Build history of the part. All positions in model axes, mm. A direction names the side the tool comes from. Round coordinates to 2 decimals unless told otherwise and drop trailing zeros. Loops run counter-clockwise (first coordinate to the right, second up) from the corner with the lowest first, then second, coordinate; pieces in that order, holes last. Notation, with made-up numbers: (-16, 58) -> (34, 58) arc R10 cw to (34, 72) -> close; hole circle Ø6 at (1, 37.25). An arc over 180 degrees is marked (long way). Put each result on its own line as item: value. Start each with the question number.
Item 1: Cut at C-C, the plane x = -4. List the corners of the cut face in (y, z) (3 decimals).
Item 2: Flat gauge pins, fed straight in: pin 1 Ø12 at (x, z) = (-22, -19.5) entering from -Y; pin 2 Ø0.5 at (y, z) = (0.5, -36.5) entering from +X; pin 3 Ø7.5 at (x, z) = (-12, -15.5) entering from +Y. Where does each tip first touch, or does it go through?
Item 3: Drill centre lines: probe 1 along X at (y, z) = (1, -55) (3 decimals); probe 2 along X at (y, z) = (4, -47.41); probe 3 along Z at (x, y) = (-11.5, 0.6) (3 decimals). Where is each one in solid material? Low to high. Write a range as [from, to].
Item 4: Cut at A-A, the plane y = 1.05. List the corners of the cut face in (x, z) (3 decimals).
Item 5: Tool access for faces 1 (the cylindrical face through (-18.156, 4.053, -35.451)), 2 (the flat face through (0, 2, -32)), 3 (the flat face through (-2.915, 1, -36)): list every direction of +Z, -Z, +X, -X, +Y, -Y with a clear straight run to the whole face (end or side of a thin tool).
Item 6: Cut at D-D, the plane x = -15.5. List the corners of the cut face in (y, z) (3 decimals), plus the area to 3 significant figures.
Item 7: Pull direction X, two halves, no side cores. Call faces 4 (the flat face through (-31, 2, -32)), 5 (the flat face through (-15, 2, 0)), 6 (the cylindrical face through (-3.044, 4.053, -20.09)): +X half, -X half, draft (parallel to the pull), parting line (faces both ways), or undercut.
Item 8: Cut at B-B, the plane z = -44. List the corners of the cut face in (x, y) (3 decimals).
Autodesk Inventor part; units mm, degrees
ref_plane "YZ Plane" through (0, 0, 0) normal (1, 0, 0) x (0, 1, 0)
ref_plane "XZ Plane" through (0, 0, 0) normal (0, 1, 0) x (-1, 0, 0)
ref_plane "XY Plane" through (0, 0, 0) normal (0, 0, 1) x (1, 0, 0)
sketch "Sketch1" plane through (0, 0, 0) normal (0, 1, 0) x (-1, 0, 0)
  line L0 (0, 0) -> (31, 0)
  line L1 (31, 0) -> (31, -64)
  line L2 (31, -64) -> (0, -64)
  line L3 (0, -64) -> (0, 0)
  line L4 (28.085, -10.96) -> (2.915, -10.96)
  line L5 (2.915, -10.96) -> (2.915, -61.085)
  line L6 (2.915, -61.085) -> (28.085, -61.085)
  line L7 (28.085, -61.085) -> (28.085, -10.96)
  line L8 (31, -43.4956) -> (28.085, -43.4956) construction
  line L9 (15.5, -61.085) -> (15.5, -64) construction
  line L10 (31, -4.16) -> (0, -4.16)
  line L11 (31, -10.96) -> (0, -10.96)
  point P0 (15.5, -10.96)
  point P1 (15.5, 0)
  dimension "d0" = 31
  dimension "d1" = 64
  dimension "d2" = 25.17
  dimension "d4" = 4.16
  dimension "d5" = 6.8
extrude "Extrusion1" add sketch "Sketch1" along normal blind 4.3
extrude "Extrusion2" cut sketch "Sketch1" along normal blind 1.75 contours L4 L7 L6 L5
sketch "Sketch2" plane through (0, 4.3, 0) normal (0, 1, 0) x (1, 0, 0)
  circle A0 centre (-15.5, 47.41) radius 12.25
  line L0 (0, 64) -> (-31, 64)
  circle A1 centre (-14.7283, 16.41) radius 12.25
  line L1 (-31, 0) -> (0, 0)
  point P0 (-15.5, 64)
  dimension "d10" = 24.5
  dimension "d11" = 4.34
  dimension "d13" = 28.66
extrude "Extrusion3" cut sketch "Sketch2" against normal blind 0.5
properties part number "ShelfLabel"
Reply:
1. outline: (0, -64) -> (4.3, -64) -> (4.3, -51.63) -> (3.8, -51.63) -> (3.8, -43.19) -> (4.3, -43.19) -> (4.3, -22.323) -> (3.8, -22.323) -> (3.8, -10.497) -> (4.3, -10.497) -> (4.3, 0) -> (0, 0) -> (0, -10.96) -> (1.75, -10.96) -> (1.75, -61.085) -> (0, -61.085) -> close
2. pin 1: stops at y = 1.75
2. pin 2: stops at x = 0
2. pin 3: stops at y = 3.8
3. probe 1: x = [-31, -28.085], [-2.915, 0]
3. probe 2: x = [-31, -27.75], [-3.25, 0]
3. probe 3: z = [-64, -61.085], [-10.96, 0]
4. outline: (-31, -64) -> (0, -64) -> (0, 0) -> (-31, 0) -> close; hole (-28.085, -61.085) -> (-2.915, -61.085) -> (-2.915, -10.96) -> (-28.085, -10.96) -> close
5. face 1: +Y
5. face 2: +Z, -Z, +X, +Y, -Y
5. face 3: -Y
6. outline: (0, -64) -> (4.3, -64) -> (4.3, -59.66) -> (3.8, -59.66) -> (3.8, -35.16) -> (4.3, -35.16) -> (4.3, -28.636) -> (3.8, -28.636) -> (3.8, -4.184) -> (4.3, -4.184) -> (4.3, 0) -> (0, 0) -> (0, -10.96) -> (1.75, -10.96) -> (1.75, -61.085) -> (0, -61.085) -> close
6. area: 163 mm^2
7. face 4: -X half
7. face 5: draft
7. face 6: undercut
8. outline: (-31, 0) -> (-28.085, 0) -> (-28.085, 1.75) -> (-2.915, 1.75) -> (-2.915, 0) -> (0, 0) -> (0, 4.3) -> (-3.734, 4.3) -> (-3.734, 3.8) -> (-27.266, 3.8) -> (-27.266, 4.3) -> (-31, 4.3) -> close
